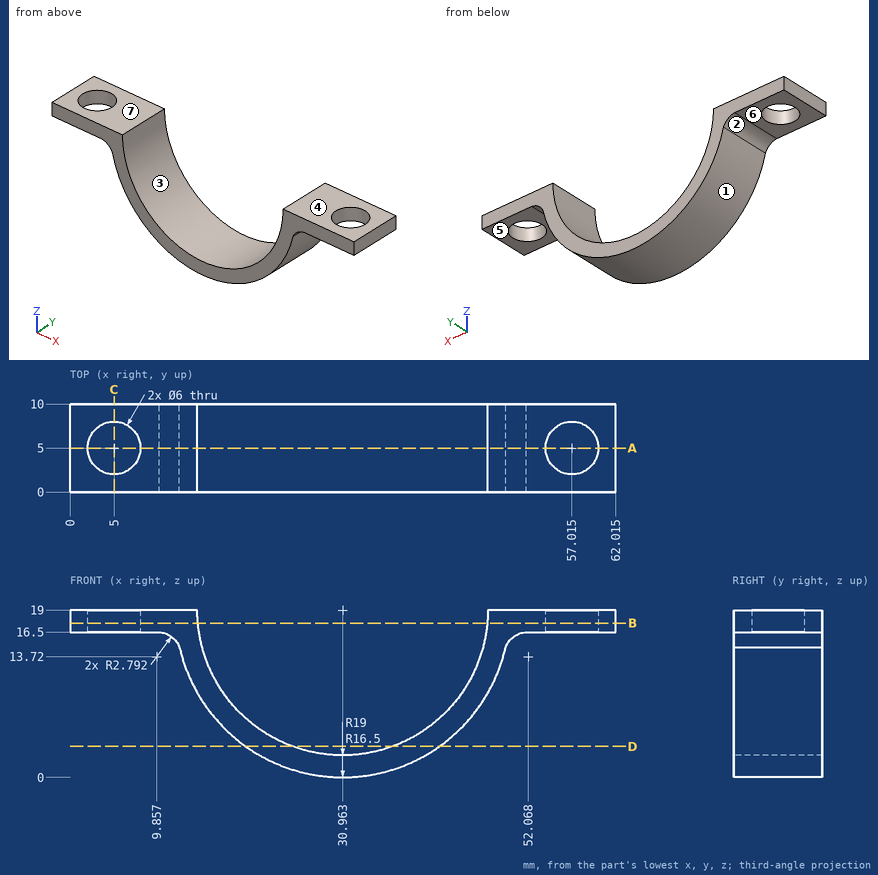
For this review, use the dimensioned drawing (mm, ordinates from the lowest corner) and the shaded views. A direction names the side the tool comes from. Give positions to 0.01 mm unless a question says otherwise; leave off trailing zeros. Write each loop counter-clockwise with the first axis right and the second up, starting at its lowest first coordinate (ties: lowest second). Pieces come first, ordered by that corner, then holes. Notation, with made-up numbers: M -2.75,1 L 37.25,1 A25 cw 37.25,23 Z; hole C 74.5,71.5 d11. An arc over 180 degrees is marked long. Answer as a JSON object with one key per item and string values. Group by question number.
Item 1: Tool access review of the marked faces 5, 6 and 7: name each direction out of +Z, -Z, +X, -X, +Y, -Y from which nothing blocks a thin tool from reaching the whole face with its end or side.
Item 2: Draft analysis for pull direction X (two halves, no side actions). For the marked faces 1, 2, 3 and 4, state which applies: +X half, -X half, draft (parallel to the pull), parting line (faces both ways), or undercut.
Item 3: For pin 1 Ø5 at (x, y) = (24, 5.5) entering from -Z; pin 2 Ø3 at (x, y) = (56.5, 6.5) entering from -Z; pin 3 Ø1.5 at (x, y) = (39.5, 1.5) entering from -Z; pin 4 Ø2 at (x, z) = (14, 8) entering from -Y, all flat-tipped, find the tip position at first contact; note any pin that passes through.
Item 4: Consider section C-C on x = 5. Write out the cut boundary in (y, z), plus the area to 3 significant figures.
Item 5: Consider section D-D on z = 3.5. Write out the cut boundary in (x, y), plus the area to 3 significant figures.
Item 6: Consider section B-B on z = 17.5. Write out the cut boundary in (x, y) (1 decimal), plus the area to 3 significant figures.
Item 7: Consider section A-A on y = 5. Write out the cut boundary in (x, z) (1 decimal).
Item 8: For probe 1 along Y at (x, z) = (5, 18); probe 2 along X at (y, z) = (8, 10) (1 decimal); probe 3 along X at (y, z) = (8.5, 8.5) (1 decimal), list the stretches that pass through material, from the lowest coordinate up. Write a range as [from, to].
Check result:
{
 "1": {"face 5": "-Z, +X, +Y, -Y", "face 6": "-Z, -X, +Y, -Y", "face 7": "+Z, +X, -X, +Y, -Y"},
 "2": {"face 1": "parting line", "face 2": "-X half", "face 3": "undercut", "face 4": "draft"},
 "3": {"pin 1": "stops at z = 0.53", "pin 2": "stops at z = 16.5", "pin 3": "stops at z = 1.67", "pin 4": "passes through"},
 "4": {"outline": "M 0,16.5 L 2,16.5 L 2,19 L 0,19 Z; M 8,16.5 L 10,16.5 L 10,19 L 8,19 Z", "area": "10.0 mm^2"},
 "5": {"outline": "M 19.97,0 L 25.31,0 L 25.31,10 L 19.97,10 Z; M 36.62,0 L 41.95,0 L 41.95,10 L 36.62,10 Z", "area": "107 mm^2"},
 "6": {"outline": "M 0,0 L 14.5,0 L 14.5,10 L 0,10 Z; M 47.4,0 L 62,0 L 62,10 L 47.4,10 Z; hole C 5,5 d6; hole C 57,5 d6", "area": "235 mm^2"},
 "7": {"outline": "M 0,16.5 L 2,16.5 L 2,19 L 0,19 Z; M 8,16.5 L 10.1,16.5 A2.8 cw 12.4,14.8 A19 ccw 49.5,14.8 A2.8 cw 51.8,16.5 L 54,16.5 L 54,19 L 47.5,19 A16.5 cw 14.5,19 L 8,19 Z; M 60,16.5 L 62,16.5 L 62,19 L 60,19 Z"},
 "8": {"probe 1": "y = [0, 2], [8, 10]", "probe 2": "x = [14.2, 17.1], [44.8, 47.7]", "probe 3": "x = [15.1, 18.2], [43.7, 46.8]"}
}
